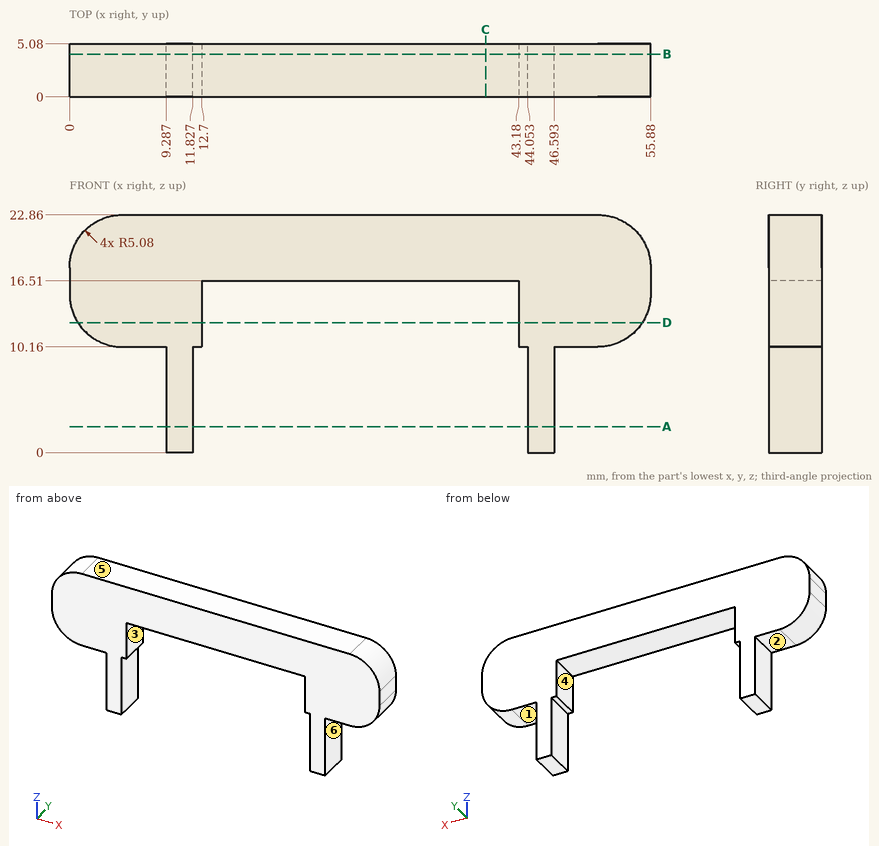
Print and shaded views of the part. All mm, measured from the part's lowest x, y and z. A direction names the side the tool comes from. Round coordinates to 2 decimals unless told otherwise and drop trailing zeros. Write each loop counter-clockwise with the first axis right and the second up, starting at its lowest first coordinate (ties: lowest second). Pieces come first, ordered by that corner, then holes. Notation, with made-up numbers: (-2, -29.75) -> (21, -29.75) arc R26 ccw to (21, -0.75) -> close; hole circle Ø4 at (71, 76.25). An arc over 180 degrees is marked (long way). Answer in a Markdown table with one row per item. Add a question column.
Item 1: Saw through at D-D, the plane z = 12.5. Write the cut outline in (x, y), then the cut area to 3 significant figures.
Item 2: Mould opens along X. For the marked faces 4, 5 and 6 say: pulls with the +X half, pulls with the -X half, needs draft (parallel to the pull), parting line crosses it, or undercut.
Item 3: Saw through at B-B, the plane y = 4.1. Write the cut outline in (x, z).
Item 4: Drill centre lines: line 1 (X direction, y = 3.7, z = 5.5); line 2 (X direction, y = 3.3, z = 16); line 3 (Z direction, x = 33.5, y = 1.6). Where is each one in solid material? Low to high. Write a range as from..to.
Item 5: Which spindle directions (+Z, -Z, +X, -X, +Y, -Y) get a long thin tool onto all of the face, cutting with end or side? Do the marked faces 1, 2 and 3. Say none if no direction does.
Item 6: Saw through at C-C, the plane x = 40. Write the cut outline in (y, z).
Item 7: Drop flat-ended pins along their axis: pin 1 Ø2 at (y, z) = (4, 10.5) entering from -X; pin 2 Ø2.5 at (y, z) = (2.5, 15) entering from +X; pin 3 Ø1 at (x, y) = (43.5, 3.5) entering from -Z; pin 4 Ø1.5 at (y, z) = (2, 3.5) entering from +X. Give the stop position or say it passes through.
Item 8: Saw through at A-A, the plane z = 2.5. Write the cut outline in (x, y).
Findings below:
| question | item | result |
|---|---|---|
| 1 | outline | (0.8, 0) -> (12.7, 0) -> (12.7, 5.08) -> (0.8, 5.08) -> close; (43.18, 0) -> (55.08, 0) -> (55.08, 5.08) -> (43.18, 5.08) -> close |
| 1 | area | 121 mm^2 |
| 2 | face 4 | undercut |
| 2 | face 5 | needs draft |
| 2 | face 6 | pulls with the +X half |
| 3 | outline | (0, 15.24) arc R5.08 ccw to (5.08, 10.16) -> (9.29, 10.16) -> (9.29, 0) -> (11.83, 0) -> (11.83, 10.16) -> (12.7, 10.16) -> (12.7, 16.51) -> (43.18, 16.51) -> (43.18, 10.16) -> (44.05, 10.16) -> (44.05, 0) -> (46.59, 0) -> (46.59, 10.16) -> (50.8, 10.16) arc R5.08 ccw to (55.88, 15.24) -> (55.88, 17.78) arc R5.08 ccw to (50.8, 22.86) -> (5.08, 22.86) arc R5.08 ccw to (0, 17.78) -> close |
| 4 | line 1 | x = 9.29..11.83, 44.05..46.59 |
| 4 | line 2 | x = 0..12.7, 43.18..55.88 |
| 4 | line 3 | z = 16.51..22.86 |
| 5 | face 1 | -Z, +X, +Y, -Y |
| 5 | face 2 | -Z, -X, +Y, -Y |
| 5 | face 3 | -Z, +Y, -Y |
| 6 | outline | (0, 16.51) -> (5.08, 16.51) -> (5.08, 22.86) -> (0, 22.86) -> close |
| 7 | pin 1 | stops at x = 1.64 |
| 7 | pin 2 | stops at x = 55.88 |
| 7 | pin 3 | stops at z = 10.16 |
| 7 | pin 4 | stops at x = 46.59 |
| 8 | outline | (9.29, 0) -> (11.83, 0) -> (11.83, 5.08) -> (9.29, 5.08) -> close; (44.05, 0) -> (46.59, 0) -> (46.59, 5.08) -> (44.05, 5.08) -> close |
